Autodesk Inventor part; units mm, degrees
ref_plane "YZ Plane" through (0, 0, 0) normal (1, 0, 0) x (0, 1, 0)
ref_plane "XZ Plane" through (0, 0, 0) normal (0, 1, 0) x (-1, 0, 0)
ref_plane "XY Plane" through (0, 0, 0) normal (0, 0, 1) x (1, 0, 0)
sketch "草圖1" plane through (0, 0, 0) normal (0, 0, 1) x (1, 0, 0)
  line L0 (0, 0) -> (-25.6572, 0) construction
  line L1 (0, 0) -> (0, 25.6407) construction
  line L2 (-20, -5.5) -> (-8.1185, -5.5)
  line L3 (25, -0.5) -> (25, 5.5)
  line L4 (25, 5.5) -> (-25, 5.5)
  line L5 (-25, 5.5) -> (-25, -0.5)
  line L6 (-25, -5.5) -> (25, 5.5) construction
  line L7 (25, -5.5) -> (-25, 5.5) construction
  arc A0 (20, -5.5) -> (25, -0.5) centre (20, -0.5) ccw
  arc A1 (-25, -0.5) -> (-20, -5.5) centre (-20, -0.5) ccw
  line L8 (-8.1185, -5.5) -> (20, -5.5)
  line L9 (7.3, 5.5) -> (7.3, 7)
  line L10 (6.8, 7.5) -> (-6.8, 7.5)
  line L11 (-7.3, 7) -> (-7.3, 5.5)
  circle A2 centre (0, 1.5) radius 2.5
  line L12 (-7.3, 7) -> (-6.8, 7.5)
  line L13 (6.8, 7.5) -> (7.3, 7)
  point P0 (7.3, 7.5)
  point P1 (-7.3, 7.5)
  dimension "d0" = 50
  dimension "d4" = 5
  dimension "d13" = 2
  dimension "d14" = 14.6
  dimension "d15" = 5
  dimension "d20" = 0.5
  dimension "d21" = 0.5
  dimension "d22" = 0.5
  dimension "d23" = 0.5
  dimension "d27" = 11
  dimension "d28" = 4
extrude "擠出1" add sketch "草圖1" along normal mid plane 8
thread "螺紋1"
equation "\"折彎半徑\" = 厚度"
equation "\"折彎離隙寬度\" = 厚度"
equation "\"折彎離隙深度\" = 0.5 * 厚度"
equation "\"轉角離隙大小\" = 4 * 厚度"
equation "\"最小剩餘\" = 2 * 厚度"
equation "\"轉移半徑\" = 折彎半徑"
equation "\"Jacobi半徑大小\" = 折彎半徑"
equation "\"間隙大小\" = 厚度"
properties part number "0 零件" material "不鏽鋼"
Can you work these out from the model? Positions are in its coordinate system, mm. A direction names the side the tool comes from. Give positions to 0.01 mm unless a question says otherwise; leave off trailing zeros. Order: outer loops, then holes, each group sorted by start corner. A loop starts at its lowest first (then second) coordinate and runs counter-clockwise, first axis right, second up. Notation, with made-up numbers: M -25,-0.5 L 1,-0.5 A37 ccw 1,36.5 Z; hole C 57,-17.5 d5. An arc over 180 degrees is marked long. Use one line per item in the form item = value. Start each with the question number.
Item 1: If we section it at C-C (y = 0.75): Write out the boundary of the cut face in (x, z), then the cut area to 3 significant figures.
Item 2: If we section it at B-B (z = 1): Write out the boundary of the cut face in (x, y), then the cut area to 3 significant figures.
Item 3: If we section it at A-A (x = 0): Write out the boundary of the cut face in (y, z).
Item 4: If I drill on line 1 along Y through (x, z) = (0, -1.5); line 2 along Y through (x, z) = (-8, -2); line 3 along Y through (x, z) = (-7, 0.75), over which ranges is the centre line in solid material (lowest first)?
Item 5: Will these pins go through, and if not, where does the flat tip stop? pin 1 Ø2.5 at (x, z) = (14.5, 1) entering from +Y; pin 2 Ø0.8 at (y, z) = (6.5, 0) entering from -X.
Item 6: If we section it at D-D (x = -15): Write out the boundary of the cut face in (y, z).
Item 7: For faces 4 (the flat face through (0, -2, -4)), 5 (the flat face through (-7.3, 6, 0)), 6 (the flat face through (16, 5.5, 0)), which set-ups out of +Z, -Z, +X, -X, +Y, -Y let a thin tool reach every point of the face, with its end or its side?
Item 8: We'd pull the mould along Y, two halves only. Please class faces 1 (the cylindrical face through (-23.5, -4.07, -0.06)), 2 (the flat face through (-16, 5.5, 0)), 3 (the cylindrical face through (-0.54, 3.94, -0.06)): +Y half, -Y half, draft (parallel to the pull), parting line (faces both ways), or undercut.
Outcome:
q1.outline = M -25,-4 L -2.38,-4 L -2.38,4 L -25,4 Z; M 2.38,-4 L 25,-4 L 25,4 L 2.38,4 Z
q1.area = 362 mm2
q2.outline = M -25,-0.5 A5 ccw -20,-5.5 L 20,-5.5 A5 ccw 25,-0.5 L 25,5.5 L 7.3,5.5 L 7.3,7 L 6.8,7.5 L -6.8,7.5 L -7.3,7 L -7.3,5.5 L -25,5.5 Z; hole C 0,1.5 d5
q2.area = 549 mm2
q3.outline = M -5.5,-4 L -1,-4 L -1,4 L -5.5,4 Z; M 4,-4 L 7.5,-4 L 7.5,4 L 4,4 Z
q4.line_1 = -5.5 to -1, 4 to 7.5
q4.line_2 = -5.5 to 5.5
q4.line_3 = -5.5 to 7.3
q5.pin_1 = 5.5
q5.pin_2 = -7.3
q6.outline = M -5.5,-4 L 5.5,-4 L 5.5,4 L -5.5,4 Z
q7.face_4 = -Z, +X, -X, +Y, -Y
q7.face_5 = +Z, -Z, -X, +Y
q7.face_6 = +Z, -Z, +X, +Y
q8.face_1 = -Y half
q8.face_2 = +Y half
q8.face_3 = undercut
